Build history of the part. All positions in model axes, mm. Face numbers are marked on the shaded views. A direction names the side the tool comes from. Coordinates: 2 decimals unless noted, no trailing zeros. Order: outer loops, then holes, each group sorted by start corner. A loop starts at its lowest first (then second) coordinate and runs counter-clockwise, first axis right, second up. Notation, with made-up numbers: (17, -2.5) - (72, -2.5) arc R36 cw to (72, 31.5) - close; hole circle Ø9 at (-25.75, 13). An arc over 180 degrees is marked (long way). One line per item, written item: value.
Autodesk Fusion 360 part; units mm, degrees
sketch "Sketch1" plane through (0, 0, 0) normal (0, 0, 1) x (1, 0, 0)
  line L0 (0, 0) -> (16, 0)
  line L1 (16, 0) -> (16, 2)
  line L2 (16, 2) -> (2, 2)
  line L3 (2, 2) -> (2, 16)
  line L4 (2, 16) -> (0, 16)
  line L5 (0, 16) -> (0, 0)
  dimension "d1" = 16
  dimension "d2" = 16
  dimension "d3" = 2
  dimension "d4" = 2
extrude "Extrude1" add sketch "Sketch1" against normal blind 46
sketch "Sketch2" plane through (0, 2, 0) normal (0, 1, 0) x (-1, 0, 0)
  line L0 (-2, 0) -> (-16, 0)
  line L1 (-16, 0) -> (-16, -46)
  line L2 (-16, -46) -> (-2, -46)
  line L3 (-2, -46) -> (-2, 0)
  line L4 (-9, -46) -> (-9, 0) construction
  line L5 (-16, -23) -> (-2, -23) construction
  circle A0 centre (-9, -15.5) radius 1.7
  circle A1 centre (-9, -30.5) radius 1.7
  dimension "d7" = 3.4
  dimension "d19" = 7.5
extrude "Extrude2" cut sketch "Sketch2" against normal blind 2 contours A0 | A1
sketch "Sketch3" plane through (2, 0, 0) normal (1, 0, 0) x (0, 0, -1)
  line L0 (0, 16) -> (0, 2)
  line L1 (0, 2) -> (46, 2)
  line L2 (46, 2) -> (46, 16)
  line L3 (46, 16) -> (0, 16)
  line L4 (23, 16) -> (23, 2) construction
  line L5 (0, 9) -> (46, 9) construction
  circle A0 centre (7, 9) radius 3.2
  line L6 (0, 12.2) -> (46, 12.2) construction
  line L7 (0, 6.2) -> (46, 6.2) construction
  line L8 (5.4508, 6.2) -> (8.5492, 6.2)
  circle A1 centre (39, 9) radius 3.2
  line L9 (40.5492, 6.2) -> (37.4508, 6.2)
  dimension "d10" = 6.4
  dimension "d11" = 6
  dimension "d12" = 16
extrude "Extrude3" cut sketch "Sketch3" against normal blind 2 contours A0 L8 | A1 L9 picked at (6.9734, 8.1997) picked at (38.4662, 7.5792)
fillet "Fillet1" radius 2 1 edges at (2, 2, -23)
fillet "Fillet2" radius 3 4 edges at (1, 16, -46) (1, 16, 0) (16, 1, 0) (16, 1, -46)
equation "d12 = ( 32 / 2 ) * 1 mm"
equation "d19 = ( 15 / 2 ) * 1 mm"
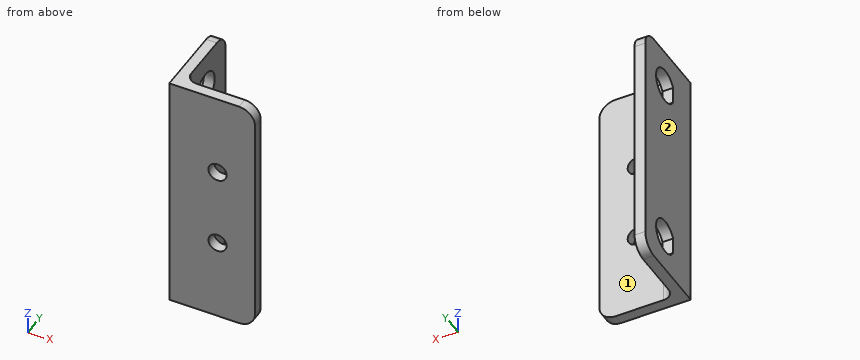
1. Probe line 1 along Z through (x, y) = (1, 9); line 2 along Y through (x, z) = (0.7, -7); line 3 along Z through (x, y) = (9, 1). List the from-to ranges inside material, lowest first.
Values found:
line 1: z = -46 to -42.2, -35.8 to -10.2, -3.8 to 0
line 2: y = 0 to 6.2, 12.2 to 16
line 3: z = -46 to -32.2, -28.8 to -17.2, -13.8 to 0
2. Band-saw the part on C-C, the plane x = 1.5. Give the cut face in (y, z).
Values found:
outline: (0, -46) - (13, -46) arc R3 ccw to (16, -43) - (16, -3) arc R3 ccw to (13, 0) - (0, 0) - close; hole (6.2, -40.55) arc R3.2 ccw (long way) to (6.2, -37.45) - close; hole (6.2, -8.55) arc R3.2 ccw (long way) to (6.2, -5.45) - close
3. Band-saw the part on A-A, the plane z = -39. Give the cut face in (x, y), and give its area (3 significant figures).
Values found:
outline: (0, 0) - (16, 0) - (16, 2) - (4, 2) arc R2 cw to (2, 4) - (2, 6.2) - (0, 6.2) - close; (0, 12.2) - (2, 12.2) - (2, 16) - (0, 16) - close
area: 48.9 mm2
4. 3-axis set-ups, long thin cutter, end or side, ignore diameter. For the marked faces 1 and 2: which of +Z, -Z, +X, -X, +Y, -Y reach the whole face in a straight line?
Values found:
face 1: +Z, -Z, +X, +Y
face 2: +Z, -Z, -X, +Y, -Y
5. Band-saw the part on D-D, the plane z = -30.5. Give the cut face in (x, y).
Values found:
outline: (0, 0) - (7.3, 0) - (7.3, 2) - (4, 2) arc R2 cw to (2, 4) - (2, 16) - (0, 16) - close; (10.7, 0) - (16, 0) - (16, 2) - (10.7, 2) - close
6. Band-saw the part on B-B, the plane y = 9. Give the cut face in (x, z), and give its area (3 significant figures).
Values found:
outline: (0, -46) - (2, -46) - (2, -42.2) - (0, -42.2) - close; (0, -35.8) - (2, -35.8) - (2, -10.2) - (0, -10.2) - close; (0, -3.8) - (2, -3.8) - (2, 0) - (0, 0) - close
area: 66.4 mm2
7. Flat gauge pins, fed straight in: P1, Ø8.5, axis at y = 9, z = -39, coming from the +X side; P2, Ø9.5, axis at x = 7, z = -26, coming from the +Y side; P3, Ø1, axis at x = 14, z = -14.5, coming from the +Y side. Where does each tip first touch, or does it go through?
Values found:
P1: stops at x = 2
P2: stops at y = 3.03
P3: stops at y = 2
